The listing builds one solid part. Answer for the finished solid, in the listing's coordinates (mm). A direction names the side the tool comes from. Round coordinates to 2 decimals unless told otherwise and drop trailing zeros. Write each loop counter-clockwise with the first axis right and the second up, starting at its lowest first coordinate (ties: lowest second). Pieces come first, ordered by that corner, then holes. Notation, with made-up numbers: (77, 81.25) - (92, 81.25) arc R21 ccw to (92, 103.25) - close; hole circle Ø10 at (7.5, -8). An arc over 180 degrees is marked (long way). Return JSON: item names as keys, results as strings. Group by question number.
(1) Find the intervals of material crossed by line 1 along Y through (x, z) = (1.05, -110); line 2 along Y through (x, z) = (3.85, -61); line 3 along Z through (x, y) = (2.2, -21), in increasing order. Write a range as [from, to].
(2) Section D-D, the plane y = -8.5 is taken. Write down the section's boundary in (x, z), then the cut area to 3 significant figures.
(3) Section C-C, the plane z = -52.5 is taken. Write down the section's boundary in (x, y), then the cut area to 3 significant figures.
(4) Each of these flat-tipped pins is pushed along its axis until it touches: pin 1 (2 mm diameter, centred on x = 0.5, y = -20, fed in from +Z); pin 2 (1.2 mm diameter, centred on x = 2.5, z = -57.5, fed in from -Y); pin 3 (3.5 mm diameter, centred on y = -35.94, z = -109.12, fed in from -X); pin 4 (2 mm diameter, centred on x = 3, z = -68, fed in from -Y). Where does it stop, or does it pass through?
(5) Section B-B, the plane x = 2.2 is taken. Write down the section's boundary in (y, z).
(6) Section A-A, the plane y = 0 is taken. Write down the section's boundary in (x, z), then the cut area to 3 significant figures.
(7) Which of the six approach directions +Z, -Z, +X, -X, +Y, -Y give full straight-line access (tool end or side, diameter ignored) to faces 4 (the flat face through (2, -10, -54)), 5 (the cylindrical face through (2, 0, -62))?
(8) Determine the mould class of faces 1 (the flat face through (2, -45.938, -109)), 2 (the cylindrical face through (2.03, 0.45, -76.39)), 3 (the flat face through (2, 0, -45.5)) for opening direction Y: +Y half, -Y half, draft (parallel to the pull), parting line (faces both ways), or undercut.
```python
from build123d import *

# Parameters (mm, degrees)
SALIENTE_EXTRUIR1_DEPTH = 4
REDONDEO1_R             = 30
CROQUIS2_R              = 1.5
CORTAR_EXTRUIR1_DEPTH   = 50
CROQUIS3_R              = 1.5
CORTAR_EXTRUIR2_DEPTH   = 10


with BuildPart() as part:
    # Croquis1 → Saliente-Extruir1 (new body)
    with BuildSketch(Plane(origin=(0, 0, 0), x_dir=(0, 0, -1), z_dir=(1, 0, 0))):
        Polygon((45.499640595, 10), (75.499640595, 10), (119.117632426, -15.938244799), (119.117632426, -45.938244799), (99.117632426, -45.938244799), (99.117632426, -27.314001558), (70.002247619, -10), (45.499640595, -10), align=None)
    extrude(amount=SALIENTE_EXTRUIR1_DEPTH)

    # Redondeo1
    redondeo1_edges = [part.edges().sort_by_distance(p)[0] for p in [
        (2, -27.314001558, -99.117632426),
        (2, -10, -70.002247619),
        (2, 10, -75.499640595),
        (2, -15.938244799, -119.117632426),
    ]]
    fillet(redondeo1_edges, radius=REDONDEO1_R)

    # Croquis2 → Cortar-Extruir1 (cut)
    with BuildSketch(Plane(origin=(4, 0, 0), x_dir=(0, 0, -1), z_dir=(1, 0, 0))):
        with Locations((60.499640595, 0)):
            Circle(CROQUIS2_R)
        with Locations((74.959961296, 0)):
            Circle(CROQUIS2_R)
    extrude(amount=-CORTAR_EXTRUIR1_DEPTH, mode=Mode.SUBTRACT)

    # Croquis3 → Cortar-Extruir2 (cut)
    with BuildSketch(Plane(origin=(4, 0, 0), x_dir=(0, 0, -1), z_dir=(1, 0, 0))):
        with Locations((109.117632426, -35.938244799)):
            Circle(CROQUIS3_R)
        with Locations((109.117632426, -20.938244799)):
            Circle(CROQUIS3_R)
    extrude(amount=-CORTAR_EXTRUIR2_DEPTH, mode=Mode.SUBTRACT)


solid = part.part
```
Working result:
{
 "1": {"line 1": "y = [-45.94, -37.15], [-34.73, -22.15], [-19.73, -11.46]", "line 2": "y = [-10, -1.41], [1.41, 10]", "line 3": "z = [-116.61, -110.62], [-107.62, -87.92]"},
 "2": {"outline": "(0, -106.43) - (4, -106.43) - (4, -45.5) - (0, -45.5) - close", "area": "244 mm^2"},
 "3": {"outline": "(0, -10) - (4, -10) - (4, 10) - (0, 10) - close", "area": "80.0 mm^2"},
 "4": {"pin 1": "stops at z = -85.12", "pin 2": "stops at y = -10", "pin 3": "stops at x = 0", "pin 4": "stops at y = -10.89"},
 "5": {"outline": "(-45.94, -119.12) - (-33, -119.12) arc R30 ccw to (-7.22, -104.45) - (5.79, -82.59) arc R30 ccw to (10, -67.25) - (10, -45.5) - (-10, -45.5) - (-10, -61.76) arc R30 cw to (-14.21, -77.09) - (-18.59, -84.45) arc R30 cw to (-44.38, -99.12) - (-45.94, -99.12) - close; hole circle Ø3 at (-35.94, -109.12); hole circle Ø3 at (-20.94, -109.12); hole circle Ø3 at (0, -74.96); hole circle Ø3 at (0, -60.5)"},
 "6": {"outline": "(0, -92.32) - (4, -92.32) - (4, -76.46) - (0, -76.46) - close; (0, -73.46) - (4, -73.46) - (4, -62) - (0, -62) - close; (0, -59) - (4, -59) - (4, -45.5) - (0, -45.5) - close", "area": "163 mm^2"},
 "7": {"face 4": "+Z, +X, -X, -Y", "face 5": "+X, -X"},
 "8": {"face 1": "-Y half", "face 2": "undercut", "face 3": "draft"}
}
